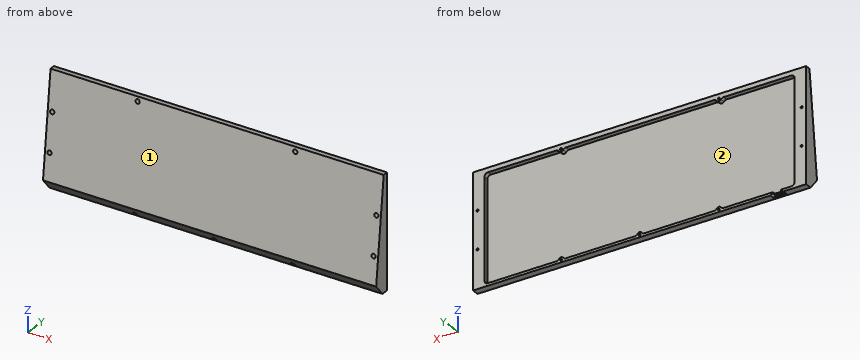
```python
from build123d import *

# Parameters (mm, degrees)
SKETCH1_W               = 390.8
SKETCH1_H               = 133.8
BOSS_EXTRUDE1_DEPTH     = 6
SKETCH2_W               = 364
SKETCH2_H               = 125.6
CUT_EXTRUDE1_DEPTH      = 5.5
BOSS_EXTRUDE3_DEPTH     = 390.8
SKETCH8_W               = 9.2
SKETCH8_H               = 3.5
CUT_EXTRUDE2_DEPTH      = 10
BOSS_EXTRUDE4_DEPTH     = 5.5
SKETCH11_W              = 15.2
SKETCH11_H              = 5.5
CUT_EXTRUDE3_DEPTH      = 1.5
CUT_EXTRUDE6_DEPTH      = 414.351517904
CUT_EXTRUDE6_DEPTH_BACK = 414.351517904
FILLET1_R               = 4
M2_CLEARANCE_HOLE1_D    = 2.4
CUT_EXTRUDE7_START      = -1
SKETCH13_R              = 2.5
CUT_EXTRUDE7_DEPTH      = 413.538863107
FILLET2_R               = 4


with BuildPart() as part:
    # Sketch1 → Boss-Extrude1 (new body)
    with BuildSketch(Plane(origin=(0, 0, 0), x_dir=(1, 0, 0), z_dir=(0, 1, 0))):
        with Locations((195.4, 66.9)):
            Rectangle(SKETCH1_W, SKETCH1_H)
    extrude(amount=BOSS_EXTRUDE1_DEPTH)

    # Sketch2 → Cut-Extrude1 (cut)
    with BuildSketch(Plane(origin=(0, 6, 0), x_dir=(1, 0, 0), z_dir=(0, 1, 0))):
        with Locations((195.4, 68.1)):
            Rectangle(SKETCH2_W, SKETCH2_H)
    extrude(amount=-CUT_EXTRUDE1_DEPTH, mode=Mode.SUBTRACT)

    # Boss-Extrude3: read off the stored shape, not the designer's step
    # Boss-Extrude3 outline → Boss-Extrude3 (add)
    with BuildSketch(Plane.YZ):
        Polygon((-15.244584391, -133.8), (0, -133.8), (0, 0), align=None)
    extrude(amount=BOSS_EXTRUDE3_DEPTH)

    # Sketch8 → Cut-Extrude2 (cut)
    with BuildSketch(Plane(origin=(0, 0, -133.8), x_dir=(-1, 0, 0), z_dir=(0, 0, -1))):
        with Locations((-34.3, 4.25)):
            Rectangle(SKETCH8_W, SKETCH8_H)
    extrude(amount=-CUT_EXTRUDE2_DEPTH, mode=Mode.SUBTRACT)

    # Sketch10 → Boss-Extrude4 (add)
    with BuildSketch(Plane(origin=(0, 0.5, 0), x_dir=(1, 0, 0), z_dir=(0, 1, 0))):
        with BuildLine():
            Line((99.5, 5.3), (105.5, 5.3))
            ThreePointArc((105.5, 5.3), (102.5, 8.3), (99.5, 5.3))
        make_face()
        with BuildLine():
            ThreePointArc((290.5, 5.3), (287.5, 8.3), (284.5, 5.3))
            Line((284.5, 5.3), (290.5, 5.3))
        make_face()
        with BuildLine():
            Line((105.5, 130.9), (99.5, 130.9))
            ThreePointArc((99.5, 130.9), (102.5, 127.9), (105.5, 130.9))
        make_face()
        with BuildLine():
            ThreePointArc((284.5, 130.9), (287.5, 127.9), (290.5, 130.9))
            Line((290.5, 130.9), (284.5, 130.9))
        make_face()
        with BuildLine():
            Line((198.4, 130.9), (192.4, 130.9))
            ThreePointArc((192.4, 130.9), (195.4, 127.9), (198.4, 130.9))
        make_face()
    extrude(amount=BOSS_EXTRUDE4_DEPTH)

    # Sketch11 → Cut-Extrude3 (cut)
    with BuildSketch(Plane(origin=(0, 0, -133.8), x_dir=(-1, 0, 0), z_dir=(0, 0, -1))):
        with Locations((-34.3, 3.25)):
            Rectangle(SKETCH11_W, SKETCH11_H)
    extrude(amount=-CUT_EXTRUDE3_DEPTH, mode=Mode.SUBTRACT)

    # Sketch12 → Cut-Extrude6 (cut, two sides: drawn at the far end of the back side and taken through both)
    with BuildSketch(Plane.ZY.offset(-CUT_EXTRUDE6_DEPTH_BACK)):
        Polygon((-133.8, -15.244584391), (-120.069803619, -13.680226114), (-133.8, -2.2), align=None)
    extrude(amount=CUT_EXTRUDE6_DEPTH + CUT_EXTRUDE6_DEPTH_BACK, mode=Mode.SUBTRACT)

    # Fillet1
    fillet1_edges = [part.edges().sort_by_distance(p)[0] for p in [
        (13.4, 3.25, -5.3),
        (13.4, 3.25, -130.9),
        (377.4, 3.25, -130.9),
        (377.4, 3.25, -5.3),
        (99.5, 3.25, -130.9),
        (105.5, 3.25, -130.9),
        (192.4, 3.25, -130.9),
        (198.4, 3.25, -130.9),
        (284.5, 3.25, -130.9),
        (290.5, 3.25, -130.9),
        (290.5, 3.25, -5.3),
        (284.5, 3.25, -5.3),
        (105.5, 3.25, -5.3),
        (99.5, 3.25, -5.3),
    ]]
    fillet(fillet1_edges, radius=FILLET1_R)

    # M2 Clearance Hole1 (through all)
    with Locations(Plane(origin=(102.5, 6, -5.3), x_dir=(0, 0, 1), z_dir=(0, 1, 0))):
        with Locations((0, 0), (-39.7, -97.2), (-83.5, -97.2), (-125.6, 0), (-125.6, 92.9), (-125.6, 185), (-83.5, 283), (-39.7, 283), (0, 185)):
            Hole(M2_CLEARANCE_HOLE1_D / 2)

    # Sketch13 → Cut-Extrude7 (cut, through all)
    with BuildSketch(Plane(origin=(0, 6, 0), x_dir=(1, 0, 0), z_dir=(0, 1, 0)).offset(CUT_EXTRUDE7_START)):
        with Locations(Location((5.3, 45, 0), (0, 0, 270))):
            Circle(SKETCH13_R)
        with Locations(Location((5.3, 88.8, 0), (0, 0, 270))):
            Circle(SKETCH13_R)
        with Locations(Location((102.5, 5.3, 0), (0, 0, 270))):
            Circle(SKETCH13_R)
        with Locations(Location((287.5, 5.3, 0), (0, 0, 270))):
            Circle(SKETCH13_R)
        with Locations(Location((385.5, 45, 0), (0, 0, 270))):
            Circle(SKETCH13_R)
        with Locations(Location((385.5, 88.8, 0), (0, 0, 270))):
            Circle(SKETCH13_R)
        with Locations(Location((287.5, 130.9, 0), (0, 0, 270))):
            Circle(SKETCH13_R)
        with Locations(Location((195.4, 130.9, 0), (0, 0, 270))):
            Circle(SKETCH13_R)
        with Locations(Location((102.5, 130.9, 0), (0, 0, 270))):
            Circle(SKETCH13_R)
    extrude(amount=-CUT_EXTRUDE7_DEPTH, mode=Mode.SUBTRACT)

    # Fillet2
    # the kernel refuses this fillet: 4 mm, written as the material it adds along each edge
    with BuildSketch(Plane(origin=(41.9, -7.306247498, -132.3), x_dir=(-1, 0, 0), z_dir=(0, 1, 0))) as fillet2_piece_1_section:
        with BuildLine():
            CenterArc((3.122498999, -4), FILLET2_R, 90, 51.317812547)
            Line((0, -1.5), (0, 0))
            Line((0, 0), (3.122498999, 0))
        make_face()
    fillet2_piece_1 = extrude(amount=21.112494996, mode=Mode.PRIVATE)
    fillet2_piece_1 = split(fillet2_piece_1, bisect_by=Plane(origin=(41.9, 2.5, -132.3), z_dir=(0, -1, 0)), keep=Keep.TOP, mode=Mode.PRIVATE)
    fillet2_piece_1 = split(fillet2_piece_1, bisect_by=Plane(origin=(41.9, -5.039151199, -130.404413264), z_dir=(0, 0.7671651518152931, 0.6414496315691656)), keep=Keep.TOP, mode=Mode.PRIVATE)
    add(fillet2_piece_1)
    with BuildSketch(Plane(origin=(41.9, -7.306247498, -132.3), x_dir=(-1, 0, 0), z_dir=(0, 1, 0))) as fillet2_piece_2_section:
        with BuildLine():
            CenterArc((3.122498999, -4), FILLET2_R, 90, 51.317812547)
            Line((0, -1.5), (0, 0))
            Line((0, 0), (3.122498999, 0))
        make_face()
    fillet2_piece_2 = extrude(amount=13.306247498, mode=Mode.PRIVATE)
    fillet2_piece_2 = split(fillet2_piece_2, bisect_by=Plane(origin=(38.9, -7.306247498, -132.3), z_dir=(1, 0, 0)), keep=Keep.TOP, mode=Mode.PRIVATE)
    fillet2_piece_2 = split(fillet2_piece_2, bisect_by=Plane(origin=(41.9, -5.039151199, -130.404413264), z_dir=(0, 0.7671651518152931, 0.6414496315691656)), keep=Keep.TOP, mode=Mode.PRIVATE)
    add(fillet2_piece_2)
    with BuildSketch(Plane(origin=(26.7, 6, -132.3), x_dir=(1, 0, 0), z_dir=(0, -1, 0))) as fillet2_piece_3_section:
        with BuildLine():
            CenterArc((3.122498999, -4), FILLET2_R, 90, 51.317812547)
            Line((0, -1.5), (0, 0))
            Line((0, 0), (3.122498999, 0))
        make_face()
    fillet2_piece_3 = extrude(amount=13.306247498, mode=Mode.PRIVATE)
    fillet2_piece_3 = split(fillet2_piece_3, bisect_by=Plane(origin=(29.7, 6, -132.3), z_dir=(-1, 0, 0)), keep=Keep.TOP, mode=Mode.PRIVATE)
    fillet2_piece_3 = split(fillet2_piece_3, bisect_by=Plane(origin=(26.7, 0.435805859, -136.952388437), z_dir=(0, 0.7671651518152931, 0.6414496315691656)), keep=Keep.TOP, mode=Mode.PRIVATE)
    add(fillet2_piece_3)
    with BuildSketch(Plane(origin=(26.7, 13.806247498, -132.3), x_dir=(1, 0, 0), z_dir=(0, -1, 0))) as fillet2_piece_4_section:
        with BuildLine():
            CenterArc((3.122498999, -4), FILLET2_R, 90, 51.317812547)
            Line((0, -1.5), (0, 0))
            Line((0, 0), (3.122498999, 0))
        make_face()
    fillet2_piece_4 = extrude(amount=21.112494996, mode=Mode.PRIVATE)
    fillet2_piece_4 = split(fillet2_piece_4, bisect_by=Plane(origin=(26.7, 2.5, -132.3), z_dir=(0, -1, 0)), keep=Keep.TOP, mode=Mode.PRIVATE)
    fillet2_piece_4 = split(fillet2_piece_4, bisect_by=Plane(origin=(26.7, 3.647745952, -140.793825689), z_dir=(0, 0.7671651518152931, 0.6414496315691656)), keep=Keep.TOP, mode=Mode.PRIVATE)
    add(fillet2_piece_4)


solid = part.part
```
Design review of the part built by this model. Coordinates are the model's own, in mm. Face numbers are marked on the shaded views. Coordinates: 2 decimals unless noted, no trailing zeros. Write each loop counter-clockwise with the first axis right and the second up, starting at its lowest first coordinate (ties: lowest second). Pieces come first, ordered by that corner, then holes. Notation, with made-up numbers: M 45.25,16 L 67.25,16 A24 ccw 67.25,34 Z; hole C 17.25,8 d6. An arc over 180 degrees is marked long. Answer as a JSON object with one key per item and string values.
Item 1: Wall thickness on probe 1 along X at (y, z) = (0.3, -5.3); probe 2 along X at (y, z) = (2, -45); probe 3 along Z at (x, y) = (102.5, 5.7): over which ranges is each line inside the solid? List them lowest first.
Outcome:
{"probe 1": "0 to 100, 105 to 285, 290 to 390.8", "probe 2": "0 to 2.8, 7.8 to 13.4, 377.4 to 383, 388 to 390.8", "probe 3": "-133.8 to -132.1, -129.7 to -127.9, -8.3 to -6.5, -4.1 to 0"}
Item 2: Insertion check: pin 1 Ø2.5 at (x, z) = (103, -6) entering from -Y; pin 2 Ø6 at (x, y) = (346, 2) entering from +Z; pin 3 Ø8 at (x, z) = (50.5, -100.5) entering from -Y; pin 4 Ø1 at (x, y) = (35, 1.5) entering from -Z. Each pin has a flat end and moves straight along its axis. Give the tip position at first contact, or say it passes through.
Outcome:
{"pin 1": "y = 5", "pin 2": "z = 0", "pin 3": "y = -11.91", "pin 4": "z = -132.3"}
Item 3: Draft analysis for pull direction X (two halves, no side actions). For the marked faces 1 and 2, state which applies: pulls with the +X half, pulls with the -X half, needs draft (parallel to the pull), parting line crosses it, or undercut.
Outcome:
{"face 1": "needs draft", "face 2": "undercut"}
Item 4: Add section C-C, the plane z = -115.5. Give the boundary of the cut face in (x, y), and give its area (3 significant figures).
Outcome:
{"outline": "M 0,-13.16 L 390.8,-13.16 L 390.8,6 L 377.4,6 L 377.4,0.5 L 13.4,0.5 L 13.4,6 L 0,6 Z", "area": "5,490 mm²"}
Item 5: Add section A-A, the plane x = 137. Give the boundary of the cut face in (y, z).
Outcome:
{"outline": "M -13.68,-120.07 L -2.2,-133.8 L 6,-133.8 L 6,-130.9 L 0.5,-130.9 L 0.5,-5.3 L 6,-5.3 L 6,0 L 0,0 Z"}
Item 6: Add section B-B, the plane z = -52. Give the boundary of the cut face in (x, y).
Outcome:
{"outline": "M 0,-5.92 L 390.8,-5.92 L 390.8,6 L 377.4,6 L 377.4,0.5 L 13.4,0.5 L 13.4,6 L 0,6 Z"}
